Here's how the part is built. I have some questions about the finished solid (model axes, mm). A direction names the side the tool comes from. Give positions to 0.01 mm unless a question says otherwise; leave off trailing zeros. Loops run counter-clockwise (first coordinate to the right, second up) from the corner with the lowest first, then second, coordinate; pieces in that order, holes last. Notation, with made-up numbers: (-19.75, -22.75) - (35.25, -22.75) arc R18 ccw to (35.25, -7.75) - close; hole circle Ø6 at (65, 18). An arc over 180 degrees is marked (long way). Use one line per item in the form item = value.
from build123d import *

# Parameters (mm, degrees)
CROQUIS1_R                       = 8
SALIENTE_EXTRUIR1_DEPTH          = 33.5
TALADRO_DE_MARGEN_PARA_M61_D     = 6.4
TALADRO_DE_MARGEN_PARA_M61_DEPTH = 20
TALADRO_DE_MARGEN_PARA_M61_TIP   = 1.922753981
TALADRO_DE_MARGEN_PARA_M62_D     = 6.4
TALADRO_DE_MARGEN_PARA_M62_DEPTH = 20
TALADRO_DE_MARGEN_PARA_M62_TIP   = 1.922753981


with BuildPart() as part:
    # Croquis1 → Saliente-Extruir1 (new body, symmetric)
    with BuildSketch(Plane(origin=(0, 0, 0), x_dir=(0, 0, -1), z_dir=(1, 0, 0))):
        Circle(CROQUIS1_R)
    extrude(amount=SALIENTE_EXTRUIR1_DEPTH, both=True)

    # Taladro de margen para M61
    with Locations(Plane.ZY.offset(33.5)):
        with Locations((0, 0)):
            Hole(TALADRO_DE_MARGEN_PARA_M61_D / 2, depth=TALADRO_DE_MARGEN_PARA_M61_DEPTH)
            with Locations((0, 0, -(TALADRO_DE_MARGEN_PARA_M61_DEPTH + TALADRO_DE_MARGEN_PARA_M61_TIP / 2))):  # 118° drill point
                Cone(0, TALADRO_DE_MARGEN_PARA_M61_D / 2, TALADRO_DE_MARGEN_PARA_M61_TIP, mode=Mode.SUBTRACT)

    # Taladro de margen para M62
    with Locations(Plane(origin=(33.5, 0, 0), x_dir=(0, 0, -1), z_dir=(1, 0, 0))):
        with Locations((0, 0)):
            Hole(TALADRO_DE_MARGEN_PARA_M62_D / 2, depth=TALADRO_DE_MARGEN_PARA_M62_DEPTH)
            with Locations((0, 0, -(TALADRO_DE_MARGEN_PARA_M62_DEPTH + TALADRO_DE_MARGEN_PARA_M62_TIP / 2))):  # 118° drill point
                Cone(0, TALADRO_DE_MARGEN_PARA_M62_D / 2, TALADRO_DE_MARGEN_PARA_M62_TIP, mode=Mode.SUBTRACT)


solid = part.part
(1) If we section it at A-A (x = 20): List the corners of the cut face in (y, z) for me, plus the area to 3 significant figures.
Geometry says:
outline = circle Ø16 at (0, 0); hole circle Ø6.4 at (0, 0)
area = 169 mm²
(2) For P1, Ø1.5, axis at x = -13, y = -0.5, coming from the +Z side; P2, Ø4, axis at x = -6, y = 3.5, coming from the -Z side; P3, Ø1, axis at x = 2.5, z = -5.5, coming from the -Y side (3 decimals), each with a flat end and sliding along its axis, tell me the tip position at first contact or that it passes through.
Geometry says:
P1 = 8
P2 = -7.86
P3 = -6.245
(3) If we section it at C-C (y = -4.5): List the corners of the cut face in (x, z) for me, plus the area to 3 significant figures.
Geometry says:
outline = (-33.5, -6.61) - (33.5, -6.61) - (33.5, 6.61) - (-33.5, 6.61) - close
area = 886 mm²
(4) If we section it at B-B (z = -4): List the corners of the cut face in (x, y) for me.
Geometry says:
outline = (-33.5, -6.93) - (33.5, -6.93) - (33.5, 6.93) - (-33.5, 6.93) - close
(5) For faces 4 (the cylindrical face through (23.36, -1.947, -2.539)), 5 (the conical face through (-11.91, -0.54, -0.12)), which set-ups out of +Z, -Z, +X, -X, +Y, -Y let a thin tool reach every point of the face, with its end or its side?
Geometry says:
face_4 = +X
face_5 = -X
(6) If we section it at D-D (x = -9): List the corners of the cut face in (y, z) for me.
Geometry says:
outline = circle Ø16 at (0, 0)
(7) If I drill on probe 1 along Y at (x, z) = (23.75, 0); probe 2 along Z at (x, y) = (27.5, -1); probe 3 along Z at (x, y) = (21, 1.5), over which ranges is the centre line in solid material (lowest first)?
Geometry says:
probe_1 = -8 to -3.2, 3.2 to 8
probe_2 = -7.94 to -3.04, 3.04 to 7.94
probe_3 = -7.86 to -2.83, 2.83 to 7.86
(8) Thinking about a two-plate mould opening in Y: for faces 1 (the flat face through (33.5, 0.1, -3.4)), 2 (the cylindrical face through (0.47, -7.81, 1.73)), 3 (the cylindrical face through (-23.36, -1.947, 2.539)), which applies, pulls with the +Y half, pulls with the -Y half, needs draft (parallel to the pull), parting line crosses it, or undercut?
Geometry says:
face_1 = needs draft
face_2 = parting line crosses it
face_3 = undercut
